The listing builds one solid part. Answer for the finished solid, in the listing's coordinates (mm). A direction names the side the tool comes from. Round coordinates to 2 decimals unless told otherwise and drop trailing zeros. Write each loop counter-clockwise with the first axis right and the second up, starting at its lowest first coordinate (ties: lowest second). Pieces come first, ordered by that corner, then holes.
from build123d import *

# Parameters (mm, degrees)
F0_W      = 20
F0_H      = 12
F1_DEPTH  = 12
F1_FACE_W = 20
F1_FACE_H = 12
F2_DEPTH  = 12


with BuildPart() as f1:
    # F0 (on Top) → F1 (new body)
    with BuildSketch(Plane.XY):
        Polygon((70, -25), (70, 25), (50, 25), (-50, 25), (-70, 25), (-70, -25), (-50, -25), (50, -25), align=None)
        with Locations((60, 31)):
            Rectangle(F0_W, F0_H)
        with Locations((60, -31)):
            Rectangle(F0_W, F0_H)
        with Locations((-60, 31)):
            Rectangle(F0_W, F0_H)
        with Locations((-60, -31)):
            Rectangle(F0_W, F0_H)
    extrude(amount=F1_DEPTH)

    # F1_face (on face) → F2 (join)
    with BuildSketch(Plane(origin=(-60, -37, 6), x_dir=(1, 0, 0), z_dir=(0, -1, 0))):
        Rectangle(F1_FACE_W, F1_FACE_H)
        with Locations((120, 0)):
            Rectangle(F1_FACE_W, F1_FACE_H)
    extrude(amount=F2_DEPTH)


solid = f1.part
1. Section B-B on z = 7.75 is taken. Determine the outline of the cut face in (x, y).
Geometry says:
outline: (-70, -49) - (-50, -49) - (-50, -25) - (50, -25) - (50, -49) - (70, -49) - (70, 37) - (50, 37) - (50, 25) - (-50, 25) - (-50, 37) - (-70, 37) - close
2. Given pin 1 (8 mm diameter, centred on x = 49.5, y = 17.5, fed in from -Z); pin 2 (3.5 mm diameter, centred on x = 9.5, z = 6.5, fed in from -Y); pin 3 (12 mm diameter, centred on x = -7.5, y = -34, fed in from -Z); pin 4 (3 mm diameter, centred on x = -4, z = 5.5, fed in from +Y), each flat-ended and moving along its own axis, determine where each tip first touches the part or whether it passes through.
Geometry says:
pin 1: stops at z = 0
pin 2: stops at y = -25
pin 3: passes through
pin 4: stops at y = 25
3. For a pull along X with two mould halves and no side action, classify faces 1 (the face through (70, -7, 6)), 2 (the face through (50, 31, 6)), 3 (the face through (-60, 37, 6)) as released by +X, released by -X, zero draft, split by the parting line, or undercut.
Geometry says:
face 1: released by +X
face 2: undercut
face 3: zero draft
4. Section C-C on x = -30.5 is taken. Determine the outline of the cut face in (y, z), plus the area to 3 significant figures.
Geometry says:
outline: (-25, 0) - (25, 0) - (25, 12) - (-25, 12) - close
area: 600 mm2
5. A tool of negligible diameter and unlimited length cuts with its end or side. For faces 4 (the face through (50, -37, 6)), 5 (the face through (-50, 31, 6)), 6 (the face through (-1, -5, 12)), from which of +Z, -Z, +X, -X, +Y, -Y can it reach the whole face along a straight path? Write none if from no direction.
Geometry says:
face 4: +Z, -Z, -Y
face 5: +Z, -Z, +Y
face 6: +Z, +X, -X, +Y, -Y
6. Straight lines are drawn through the part: line 1 along X through (y, z) = (-27, 5.25); line 2 along Y through (x, z) = (32, 9). For each, find the intervals that lie inside material, in ascending order.
Geometry says:
line 1: x = -70 to -50, 50 to 70
line 2: y = -25 to 25
7. Section A-A on y = -28 is taken. Determine the outline of the cut face in (x, z), plus the area to 3 significant figures.
Geometry says:
outline: (-70, 0) - (-50, 0) - (-50, 12) - (-70, 12) - close; (50, 0) - (70, 0) - (70, 12) - (50, 12) - close
area: 480 mm2
